Build history of the part. All positions in model axes, mm. Coordinates: 2 decimals unless noted, no trailing zeros. Order: outer loops, then holes, each group sorted by start corner. A loop starts at its lowest first (then second) coordinate and runs counter-clockwise, first axis right, second up. Notation, with made-up numbers: (70, 15) - (128, 15) arc R8 cw to (128, 23) - close; hole circle Ø10 at (81.25, 65). An arc over 180 degrees is marked (long way). One line per item, written item: value.
from build123d import *

# Parameters (mm, degrees)
SKICA1_W                 = 426.5
SKICA1_H                 = 40
P_IDAT_VYSUNUT_M1_DEPTH  = 2.4
SKICA2_W                 = 423.2
SKICA2_H                 = 36.8
P_IDAT_VYSUNUT_M2_DEPTH  = 1.4
ZAOBLIT1_R               = 1.5
ZAOBLIT2_R               = 0.5
ODEBRAT_VYSUNUT_M1_DEPTH = 215.199258869


with BuildPart() as part:
    # Skica1 → Přidat vysunutím1 (new body)
    with BuildSketch(Plane.XY):
        Rectangle(SKICA1_W, SKICA1_H)
    extrude(amount=P_IDAT_VYSUNUT_M1_DEPTH)

    # Skica2 → Přidat vysunutím2 (add)
    with BuildSketch(Plane.XY.offset(2.4)):
        Rectangle(SKICA2_W, SKICA2_H)
    extrude(amount=P_IDAT_VYSUNUT_M2_DEPTH)

    # Zaoblit1
    zaoblit1_edges = [part.edges().sort_by_distance(p)[0] for p in [
        (-213.25, 20, 1.2),
        (213.25, 20, 1.2),
        (213.25, -20, 1.2),
        (-213.25, -20, 1.2),
    ]]
    fillet(zaoblit1_edges, radius=ZAOBLIT1_R)

    # Zaoblit2
    zaoblit2_edges = [part.edges().sort_by_distance(p)[0] for p in [
        (211.6, -18.4, 3.1),
        (211.6, 18.4, 3.1),
        (-211.6, 18.4, 3.1),
        (-211.6, -18.4, 3.1),
    ]]
    fillet(zaoblit2_edges, radius=ZAOBLIT2_R)

    # Skica3 → Odebrat vysunutím1 (cut, through all)
    with BuildSketch(Plane.XY.offset(2.4)):
        with BuildLine():
            Line((0, -19), (-10, -19))
            ThreePointArc((-10, -19), (-10.292893219, -19.707106781), (-11, -20))
            Line((-11, -20), (-11, -20.116946074))
            Line((-11, -20.116946074), (11, -20.116946074))
            Line((11, -20.116946074), (11, -20))
            ThreePointArc((11, -20), (10.292893219, -19.707106781), (10, -19))
            Line((10, -19), (0, -19))
        make_face()
    extrude(amount=-ODEBRAT_VYSUNUT_M1_DEPTH, mode=Mode.SUBTRACT)


solid = part.part
1. Flat gauge pins, fed straight in: P1, Ø1.1, axis at x = -93, z = 3, coming from the +Y side; P2, Ø0.7, axis at x = 86, z = 3, coming from the -Y side; P3, Ø1, axis at y = -14, z = 3.5, coming from the +X side; P4, Ø6, axis at x = -29, y = -5.5, coming from the -Z side. Where does each tip first touch, or does it go through?
Values found:
P1: stops at y = 18.4
P2: stops at y = -18.4
P3: stops at x = 211.6
P4: stops at z = 0
2. Probe line 1 along Y through (x, z) = (-32, 2.8); line 2 along X through (y, z) = (0, 2.7). List the from-to ranges inside material, lowest first.
Values found:
line 1: y = -18.4 to 18.4
line 2: x = -211.6 to 211.6
3. Band-saw the part on A-A, the plane x = 94. Give the cut face in (y, z).
Values found:
outline: (-20, 0) - (20, 0) - (20, 2.4) - (18.4, 2.4) - (18.4, 3.8) - (-18.4, 3.8) - (-18.4, 2.4) - (-20, 2.4) - close
4. Band-saw the part on B-B, the plane z = 3. Give the cut face in (x, y).
Values found:
outline: (-211.6, -17.9) arc R0.5 ccw to (-211.1, -18.4) - (211.1, -18.4) arc R0.5 ccw to (211.6, -17.9) - (211.6, 17.9) arc R0.5 ccw to (211.1, 18.4) - (-211.1, 18.4) arc R0.5 ccw to (-211.6, 17.9) - close
